Model file for the job. Use its own axes, mm. A direction names the side the tool comes from. Coordinates: 2 decimals unless noted, no trailing zeros. Write each loop counter-clockwise with the first axis right and the second up, starting at its lowest first coordinate (ties: lowest second). Pieces come first, ordered by that corner, then holes.
Q1. Band-saw the part on B-B, the plane x = -4. Write the cut outline in (y, z), plus the area to 3 significant figures.
Q2. Pin check, flat tips, straight feed: P1, Ø5, axis at y = -3.5, z = -6.5, coming from the -X side; P2, Ø2, axis at y = 1.5, z = -12.5, coming from the +X side; P3, Ø8.5, axis at x = 4, z = -15, coming from the -Y side. Stop position of each tip, or through.
Q3. Drill centre lines: probe 1 along X at (y, z) = (-5.5, -4.5); probe 2 along X at (y, z) = (-10, 2.5). Where is each one in solid material? Low to high.
Q4. Which spindle directions (+Z, -Z, +X, -X, +Y, -Y) get a long thin tool onto all of the face, cutting with end or side? Do faces 1 (the cylindrical face through (-9.93, -9.9, -11.83)), 2 (the cylindrical face through (11.359, -11.297, 1.385)), 3 (the flat face through (11, 0, 0)). Say none if no direction does.
Q5. Band-saw the part on D-D, the plane z = -10.75. Write the cut outline in (x, y), plus the area to 3 significant figures.
Q6. Band-saw the part on A-A, the plane z = 1.5. Write the cut outline in (x, y), plus the area to 3 significant figures.
Autodesk Inventor part; units mm, degrees
ref_plane "YZ Plane" through (0, 0, 0) normal (1, 0, 0) x (0, 1, 0)
ref_plane "XZ Plane" through (0, 0, 0) normal (0, 1, 0) x (-1, 0, 0)
ref_plane "XY Plane" through (0, 0, 0) normal (0, 0, 1) x (1, 0, 0)
sketch "Sketch1" plane through (0, 0, 0) normal (0, 0, 1) x (1, 0, 0)
  line L0 (8.5, 10.5) -> (-8.5, 10.5)
  line L1 (8.5, 10.5) -> (-8.5, 10.5)
  arc A0 (10.5, 8.5) -> (8.5, 10.5) centre (8.5, 8.5) ccw
  line L2 (10.5, -8.5) -> (10.5, 8.5)
  arc A1 (8.5, -10.5) -> (10.5, -8.5) centre (8.5, -8.5) ccw
  line L3 (-8.5, -10.5) -> (8.5, -10.5)
  arc A2 (-10.5, -8.5) -> (-8.5, -10.5) centre (-8.5, -8.5) ccw
  line L4 (-10.5, 8.5) -> (-10.5, -8.5)
  arc A3 (-8.5, 10.5) -> (-10.5, 8.5) centre (-8.5, 8.5) ccw
  line L5 (-12.5, -8.5) -> (-12.5, 8.5)
  arc A4 (-12.5, -8.5) -> (-8.5, -12.5) centre (-8.5, -8.5) ccw
  line L6 (8.5, -12.5) -> (-8.5, -12.5)
  arc A5 (8.5, -12.5) -> (12.5, -8.5) centre (8.5, -8.5) ccw
  line L7 (12.5, 8.5) -> (12.5, -8.5)
  arc A6 (12.5, 8.5) -> (8.5, 12.5) centre (8.5, 8.5) ccw
  line L8 (-8.5, 12.5) -> (8.5, 12.5)
  arc A7 (-8.5, 12.5) -> (-12.5, 8.5) centre (-8.5, 8.5) ccw
  point P0 (0, 0)
extrude "Extrusion1" add sketch "Sketch1" against normal blind 25 contours A0 L2 A1 L3 A2 L4 A3 L0
sketch "Sketch2" plane through (0, 0, 0) normal (0, 0, 1) x (1, 0, 0)
  line L0 (8.5, 10.5) -> (-8.5, 10.5)
  arc A0 (10.5, 8.5) -> (8.5, 10.5) centre (8.5, 8.5) ccw
  line L1 (10.5, -8.5) -> (10.5, 8.5)
  arc A1 (8.5, -10.5) -> (10.5, -8.5) centre (8.5, -8.5) ccw
  line L2 (-8.5, -10.5) -> (8.5, -10.5)
  arc A2 (-10.5, -8.5) -> (-8.5, -10.5) centre (-8.5, -8.5) ccw
  line L3 (-10.5, 8.5) -> (-10.5, -8.5)
  arc A3 (-8.5, 10.5) -> (-10.5, 8.5) centre (-8.5, 8.5) ccw
  line L4 (-12.5, -8.5) -> (-12.5, 8.5)
  arc A4 (-12.5, -8.5) -> (-8.5, -12.5) centre (-8.5, -8.5) ccw
  line L5 (8.5, -12.5) -> (-8.5, -12.5)
  arc A5 (8.5, -12.5) -> (12.5, -8.5) centre (8.5, -8.5) ccw
  line L6 (12.5, 8.5) -> (12.5, -8.5)
  arc A6 (12.5, 8.5) -> (8.5, 12.5) centre (8.5, 8.5) ccw
  line L7 (-8.5, 12.5) -> (8.5, 12.5)
  arc A7 (-8.5, 12.5) -> (-12.5, 8.5) centre (-8.5, 8.5) ccw
  point P0 (0, 0)
extrude "Extrusion2" add sketch "Sketch2" along normal blind 4 contours A0 L1 A1 L2 A2 L3 A3 L0 | L4 A7 L7 A6 L6 A5 L5 A4
chamfer "Chamfer1" distance 1 angle 45 8 edges at (0, 10.5, -25) (9.9142, 9.9142, -25) (10.5, 0, -25) (9.9142, -9.9142, -25) (0, -10.5, -25) (-9.9142, -9.9142, -25) (-10.5, 0, -25) (-9.9142, 9.9142, -25)
chamfer "Chamfer2" distance 1.5 angle 45 8 edges at (0, 12.5, 4) (-11.3284, 11.3284, 4) (-12.5, 0, 4) (-11.3284, -11.3284, 4) (0, -12.5, 4) (11.3284, -11.3284, 4) (12.5, 0, 4) (11.3284, 11.3284, 4)
chamfer "Chamfer3" distance 0.3 angle 45 8 edges at (0, 12.5, 0) (11.3284, 11.3284, 0) (12.5, 0, 0) (11.3284, -11.3284, 0) (0, -12.5, 0) (-11.3284, -11.3284, 0) (-12.5, 0, 0) (-11.3284, 11.3284, 0)
properties part number "nút nhựa bit hộp thép 25x25"
Answer sheet:
1. outline: (-12.5, 0.3) - (-12.2, 0) - (-10.5, 0) - (-10.5, -24) - (-9.5, -25) - (9.5, -25) - (10.5, -24) - (10.5, 0) - (12.2, 0) - (12.5, 0.3) - (12.5, 2.5) - (11, 4) - (-11, 4) - (-12.5, 2.5) - close
1. area: 622 mm2
2. P1: stops at x = -10.5
2. P2: stops at x = 10.5
2. P3: stops at y = -10.5
3. probe 1: x = -10.5 to 10.5
3. probe 2: x = -12.21 to 12.21
4. face 1: -Z, -X, -Y
4. face 2: +Z, -Z, +X, -Y
4. face 3: -Z
5. outline: (-10.5, -8.5) arc R2 ccw to (-8.5, -10.5) - (8.5, -10.5) arc R2 ccw to (10.5, -8.5) - (10.5, 8.5) arc R2 ccw to (8.5, 10.5) - (-8.5, 10.5) arc R2 ccw to (-10.5, 8.5) - close
5. area: 438 mm2
6. outline: (-12.5, -8.5) arc R4 ccw to (-8.5, -12.5) - (8.5, -12.5) arc R4 ccw to (12.5, -8.5) - (12.5, 8.5) arc R4 ccw to (8.5, 12.5) - (-8.5, 12.5) arc R4 ccw to (-12.5, 8.5) - close
6. area: 611 mm2
